The figure shows three views and two pictorial views of one solid part (mm, origin at its lowest corner). Answer the questions. A direction names the side the tool comes from. Coordinates: 2 decimals unless noted, no trailing zeros. Order: outer loops, then holes, each group sorted by start corner. A loop starts at its lowest first (then second) coordinate and runs counter-clockwise, first axis right, second up. Notation, with made-up numbers: M -32.5,-30.5 L 10.5,-30.5 A22 cw 10.5,3.5 Z; hole C -26,58.25 d9. An arc over 180 degrees is marked long. Answer in a Markdown table with one row per item. Add a question column.
Item 1: The mould has two halves that part along X. Classify the marked faces 4, 5, 6 and 7: released by +X, released by -X, zero draft, split by the parting line, or undercut.
Item 2: The part is cut by section D-D (z = 11). Write down the section's boundary in (x, y), then the cut area to 3 significant figures.
Item 3: Flat-ended cylindrical pins translate along their axes: pin 1 Ø8 at (x, y) = (27.5, 7.5) entering from -Z; pin 2 Ø9 at (x, y) = (17.5, 16.5) entering from -Z; pin 3 Ø0.6 at (x, z) = (13.5, 29.5) entering from +Y; pin 4 Ø2 at (y, z) = (17.5, 30.5) entering from -X. Find the tip coordinate at first contact, or state that the pin passes through.
Item 4: Consider line 1 (Y direction, x = 16, z = 17.25); line 2 (Y direction, x = 16, z = 6.5); line 3 (Y direction, x = 18.5, z = 6.5). Determine where each line is inside the solid, lowest interval first. Write a range as from..to.
Item 5: Which of the six approach directions +Z, -Z, +X, -X, +Y, -Y give full straight-line access (tool end or side, diameter ignored) to the marked faces 1, 2 and 3?
Item 6: The part is cut by section A-A (x = 16). Write down the section's boundary in (y, z), then the cut area to 3 significant figures.
Item 7: The part is cut by section B-B (z = 21). Write down the section's boundary in (x, y).
Item 8: The part is cut by section C-C (y = 23). Write down the section's boundary in (x, z), then the cut area to 3 significant figures.
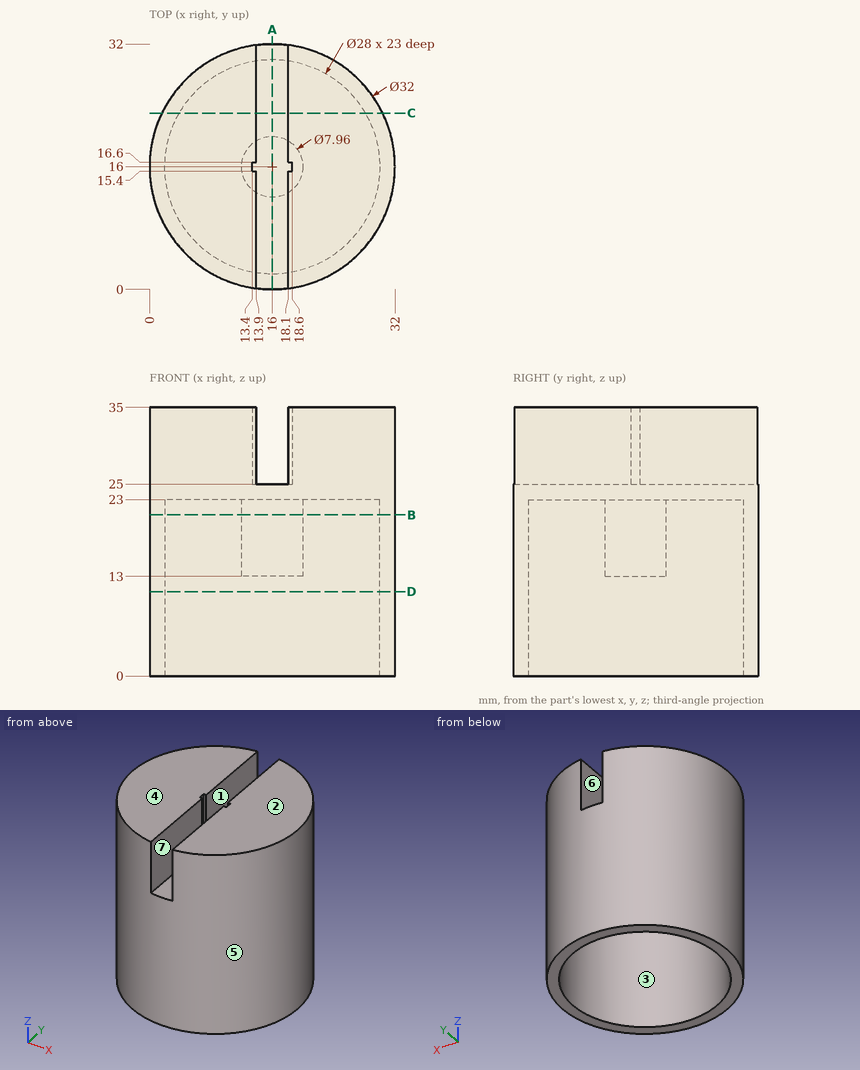
Reply:
| question | item | result |
|---|---|---|
| 1 | face 4 | zero draft |
| 1 | face 5 | split by the parting line |
| 1 | face 6 | undercut |
| 1 | face 7 | undercut |
| 2 | outline | C 16,16 d32; hole C 16,16 d28 |
| 2 | area | 188 mm2 |
| 3 | pin 1 | stops at z = 0 |
| 3 | pin 2 | stops at z = 13 |
| 3 | pin 3 | stops at y = 31.85 |
| 3 | pin 4 | stops at x = 0.01 |
| 4 | line 1 | y = 0..2, 12.02..19.98, 30..32 |
| 4 | line 2 | y = 0..2, 30..32 |
| 4 | line 3 | y = 0.2..2.23, 29.77..31.8 |
| 5 | face 1 | +Z, +Y, -Y |
| 5 | face 2 | +Z, +X, -X, +Y, -Y |
| 5 | face 3 | -Z |
| 6 | outline | M 0,0 L 2,0 L 2,23 L 12.02,23 L 12.02,13 L 19.98,13 L 19.98,23 L 30,23 L 30,0 L 32,0 L 32,25 L 0,25 Z |
| 6 | area | 236 mm2 |
| 7 | outline | C 16,16 d32; C 16,16 d7.96; hole C 16,16 d28 |
| 8 | outline | M 1.61,0 L 3.88,0 L 3.88,23 L 28.12,23 L 28.12,0 L 30.39,0 L 30.39,35 L 18.1,35 L 18.1,25 L 13.9,25 L 13.9,35 L 1.61,35 Z |
| 8 | area | 407 mm2 |
